The listing builds one solid part. Answer for the finished solid, in the listing's coordinates (mm). Face numbers are marked on the shaded views. Coordinates: 2 decimals unless noted, no trailing zeros. Write each loop counter-clockwise with the first axis right and the second up, starting at its lowest first coordinate (ties: lowest second). Pieces come first, ordered by that corner, then holes.
(1) The part is cut by section B-B on x = 7.75. Determine the outline of the cut face in (y, z), plus the area to 3 significant figures.
(2) The part is cut by section C-C on x = 0. Determine the outline of the cut face in (y, z), plus the area to 3 significant figures.
(3) For a pull along Z with two mould halves and no side action, classify the marked faces 1 and 2 as +Z half, -Z half, draft (parallel to the pull), parting line (faces both ways), or undercut.
(4) Given P1, Ø6, axis at x = -9, y = 13, coming from the -Z side, flat-ended and moving along its own axis, determine where the tip first touches the part or whether it passes through.
(5) Straight lines are drawn through the part: line 1 (Y direction, x = -15, z = 0.05); line 2 (Y direction, x = -8, z = 0.05); line 3 (Y direction, x = 7, z = 0.3). For each, find the intervals that lie inside material, in ascending order.
(6) The part is cut by section D-D on y = -6.5. Determine the outline of the cut face in (x, z), plus the area to 3 significant figures.
(7) The part is cut by section A-A on y = 0. Determine the outline of the cut face in (x, z) (3 decimals), plus the area to 3 significant figures.
from build123d import *

# Parameters (mm, degrees)
SKETCH1_R           = 25.4
SKETCH1_R_2         = 1.5
SKETCH1_R_3         = 13.25
BOSS_EXTRUDE1_DEPTH = 0.396875


with BuildPart() as part:
    # Sketch1 → Boss-Extrude1 (new body)
    with BuildSketch(Plane.XY):
        Circle(SKETCH1_R)
        with Locations((-15.5, 0)):
            Circle(SKETCH1_R_2, mode=Mode.SUBTRACT)
        with Locations((-7.75, 13.423393759)):
            Circle(SKETCH1_R_2, mode=Mode.SUBTRACT)
        with Locations((7.75, 13.423393759)):
            Circle(SKETCH1_R_2, mode=Mode.SUBTRACT)
        with Locations((15.5, 0)):
            Circle(SKETCH1_R_2, mode=Mode.SUBTRACT)
        with Locations((7.75, -13.423393759)):
            Circle(SKETCH1_R_2, mode=Mode.SUBTRACT)
        with Locations((-7.75, -13.423393759)):
            Circle(SKETCH1_R_2, mode=Mode.SUBTRACT)
        Circle(SKETCH1_R_3, mode=Mode.SUBTRACT)
        with BuildLine():
            Line((-1.584648919, 17.930111204), (-1.584648919, 22.168435055))
            ThreePointArc((-1.584648919, 22.168435055), (-11.1125, 19.247414599), (-18.406103461, 12.456563747))
            Line((-18.406103461, 12.456563747), (-14.735607336, 10.337401822))
            ThreePointArc((-14.735607336, 10.337401822), (-9, 15.588457268), (-1.584648919, 17.930111204))
        make_face(mode=Mode.SUBTRACT)
        with BuildLine():
            Line((1.584648919, 17.930111204), (1.584648919, 22.168435055))
            ThreePointArc((1.584648919, 22.168435055), (11.1125, 19.247414599), (18.406103461, 12.456563747))
            Line((18.406103461, 12.456563747), (14.735607336, 10.337401822))
            ThreePointArc((14.735607336, 10.337401822), (9, 15.588457268), (1.584648919, 17.930111204))
        make_face(mode=Mode.SUBTRACT)
        with BuildLine():
            Line((16.320256255, 7.592709383), (19.990752379, 9.711871308))
            ThreePointArc((19.990752379, 9.711871308), (22.225, 0), (19.990752379, -9.711871308))
            Line((19.990752379, -9.711871308), (16.320256255, -7.592709383))
            ThreePointArc((16.320256255, -7.592709383), (18, 0), (16.320256255, 7.592709383))
        make_face(mode=Mode.SUBTRACT)
        with BuildLine():
            Line((-16.320256255, 7.592709383), (-19.990752379, 9.711871308))
            ThreePointArc((-19.990752379, 9.711871308), (-22.225, 0), (-19.990752379, -9.711871308))
            Line((-19.990752379, -9.711871308), (-16.320256255, -7.592709383))
            ThreePointArc((-16.320256255, -7.592709383), (-18, 0), (-16.320256255, 7.592709383))
        make_face(mode=Mode.SUBTRACT)
        with BuildLine():
            Line((-14.735607336, -10.337401822), (-18.406103461, -12.456563747))
            ThreePointArc((-18.406103461, -12.456563747), (-11.1125, -19.247414599), (-1.584648919, -22.168435055))
            Line((-1.584648919, -22.168435055), (-1.584648919, -17.930111204))
            ThreePointArc((-1.584648919, -17.930111204), (-9, -15.588457268), (-14.735607336, -10.337401822))
        make_face(mode=Mode.SUBTRACT)
        with BuildLine():
            Line((1.584648919, -17.930111204), (1.584648919, -22.168435055))
            ThreePointArc((1.584648919, -22.168435055), (11.1125, -19.247414599), (18.406103461, -12.456563747))
            Line((18.406103461, -12.456563747), (14.735607336, -10.337401822))
            ThreePointArc((14.735607336, -10.337401822), (9, -15.588457268), (1.584648919, -17.930111204))
        make_face(mode=Mode.SUBTRACT)
    extrude(amount=BOSS_EXTRUDE1_DEPTH)


solid = part.part
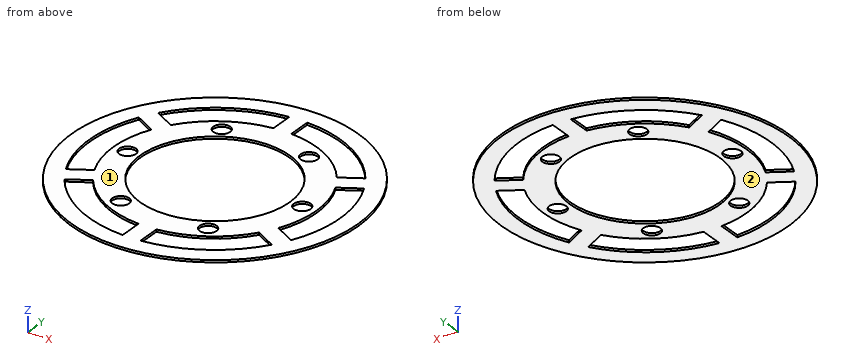
Model answer:
1. outline: (-24.19, 0) - (-20.83, 0) - (-20.83, 0.4) - (-24.19, 0.4) - close; (-16.25, 0) - (-14.92, 0) - (-14.92, 0.4) - (-16.25, 0.4) - close; (-11.92, 0) - (-10.75, 0) - (-10.75, 0.4) - (-11.92, 0.4) - close; (10.75, 0) - (11.92, 0) - (11.92, 0.4) - (10.75, 0.4) - close; (14.92, 0) - (16.25, 0) - (16.25, 0.4) - (14.92, 0.4) - close; (20.83, 0) - (24.19, 0) - (24.19, 0.4) - (20.83, 0.4) - close
1. area: 4.65 mm2
2. outline: (-25.4, 0) - (-13.25, 0) - (-13.25, 0.4) - (-25.4, 0.4) - close; (13.25, 0) - (25.4, 0) - (25.4, 0.4) - (13.25, 0.4) - close
2. area: 9.64 mm2
3. face 1: +Z half
3. face 2: -Z half
4. P1: stops at z = 0
5. line 1: y = -20.5 to -16.4, -10.49 to -1.41, 1.41 to 10.49, 16.4 to 20.5
5. line 2: y = -24.11 to -20.74, -16.12 to -14.9, -11.94 to -10.56, 10.56 to 11.94, 14.9 to 16.12, 20.74 to 24.11
5. line 3: y = -24.42 to -21.09, -16.58 to -14.72, -12.12 to -11.25, 11.25 to 12.12, 14.72 to 16.58, 21.09 to 24.42
6. outline: (-24.55, 0) - (-21.25, 0) - (-21.25, 0.4) - (-24.55, 0.4) - close; (-16.79, 0) - (-11.55, 0) - (-11.55, 0.4) - (-16.79, 0.4) - close; (11.55, 0) - (16.79, 0) - (16.79, 0.4) - (11.55, 0.4) - close; (21.25, 0) - (24.55, 0) - (24.55, 0.4) - (21.25, 0.4) - close
6. area: 6.78 mm2
7. outline: (-25.4, 0) - (-22.225, 0) - (-22.225, 0.397) - (-25.4, 0.397) - close; (-18, 0) - (-17, 0) - (-17, 0.397) - (-18, 0.397) - close; (-14, 0) - (-13.25, 0) - (-13.25, 0.397) - (-14, 0.397) - close; (13.25, 0) - (14, 0) - (14, 0.397) - (13.25, 0.397) - close; (17, 0) - (18, 0) - (18, 0.397) - (17, 0.397) - close; (22.225, 0) - (25.4, 0) - (25.4, 0.397) - (22.225, 0.397) - close
7. area: 3.91 mm2
